Could you check a few things on this model? Use its own coordinates, in mm. Give positions to 0.01 mm unless a question says otherwise; leave off trailing zeros. Loops run counter-clockwise (first coordinate to the right, second up) from the corner with the lowest first, then second, coordinate; pieces in that order, holes last. Notation, with made-up numbers: (70, 49) - (111, 49) arc R11 ccw to (111, 59) - close; hole circle Ø8 at (-16, 79). An arc over 180 degrees is marked (long way). Write each question's results on one line, items separated by ' | '. Start each with the question number.
(1) Suppose I cut it at A-A (y = 160). Please give me the cut outline in (x, z), and give its area (3 significant figures).
(2) If we mould it in two halves opening along X, with no side actions, what happens to faces 1 (the face through (12.35, 77.07, 4.93)), 2 (the face through (99, 101, 0)), 3 (the face through (0, 99, 5)), 4 (the face through (162.86, 13.9, 4.93))? For each: released by +X, released by -X, zero draft, split by the parting line, or undercut.
(3) Suppose I cut it at C-C (y = 100). Please give me the cut outline in (x, z).
(4) Suppose I cut it at B-B (x = 13). Please give me the cut outline in (y, z), and give its area (3 significant figures).
(5) I need wall thicknesses on line 1 (Y direction, x = 160, z = 4); line 2 (Y direction, x = 13, z = 3); line 3 (Y direction, x = 186, z = 2.75). Which ranges of each line are inside material? Lowest first, please.
from build123d import *

# Parameters (mm, degrees)
SKETCH_W   = 200
SKETCH_H   = 200
SKETCH_R   = 15
SKETCH_R_2 = 3
PAD_DEPTH  = 10
FILLET_R   = 3


with BuildPart() as part:
    # Sketch → Pad (new body)
    with BuildSketch(Plane.XY):
        with Locations((100, 100)):
            Rectangle(SKETCH_W, SKETCH_H)
        with Locations((136, 100)):
            Circle(SKETCH_R, mode=Mode.SUBTRACT)
        with Locations((118.32233, 117.67767)):
            Circle(SKETCH_R_2, mode=Mode.SUBTRACT)
        with Locations((153.67767, 117.67767)):
            Circle(SKETCH_R_2, mode=Mode.SUBTRACT)
        with Locations((118.32233, 82.32233)):
            Circle(SKETCH_R_2, mode=Mode.SUBTRACT)
        with Locations((153.67767, 82.32233)):
            Circle(SKETCH_R_2, mode=Mode.SUBTRACT)
        with Locations((40, 13)):
            Circle(SKETCH_R_2, mode=Mode.SUBTRACT)
        with Locations((160, 13)):
            Circle(SKETCH_R_2, mode=Mode.SUBTRACT)
        with Locations((80, 13)):
            Circle(SKETCH_R_2, mode=Mode.SUBTRACT)
        with Locations((120, 13)):
            Circle(SKETCH_R_2, mode=Mode.SUBTRACT)
        with Locations((40, 187)):
            Circle(SKETCH_R_2, mode=Mode.SUBTRACT)
        with Locations((80, 187)):
            Circle(SKETCH_R_2, mode=Mode.SUBTRACT)
        with Locations((120, 187)):
            Circle(SKETCH_R_2, mode=Mode.SUBTRACT)
        with Locations((160, 187)):
            Circle(SKETCH_R_2, mode=Mode.SUBTRACT)
        with Locations((13, 160)):
            Circle(SKETCH_R_2, mode=Mode.SUBTRACT)
        with Locations((13, 120)):
            Circle(SKETCH_R_2, mode=Mode.SUBTRACT)
        with Locations((13, 80)):
            Circle(SKETCH_R_2, mode=Mode.SUBTRACT)
        with Locations((13, 40)):
            Circle(SKETCH_R_2, mode=Mode.SUBTRACT)
        with Locations((187, 160)):
            Circle(SKETCH_R_2, mode=Mode.SUBTRACT)
        with Locations((187, 120)):
            Circle(SKETCH_R_2, mode=Mode.SUBTRACT)
        with Locations((187, 80)):
            Circle(SKETCH_R_2, mode=Mode.SUBTRACT)
        with Locations((187, 40)):
            Circle(SKETCH_R_2, mode=Mode.SUBTRACT)
    extrude(amount=PAD_DEPTH)

    # Fillet
    fillet_edges = [part.edges().sort_by_distance(p)[0] for p in [
        (0, 0, 5),
        (200, 0, 5),
        (0, 200, 5),
        (200, 200, 5),
    ]]
    fillet(fillet_edges, radius=FILLET_R)


solid = part.part
Output values:
1) outline: (0, 0) - (10, 0) - (10, 10) - (0, 10) - close; (16, 0) - (184, 0) - (184, 10) - (16, 10) - close; (190, 0) - (200, 0) - (200, 10) - (190, 10) - close | area: 1,880 mm2
2) face 1: undercut | face 2: zero draft | face 3: released by -X | face 4: undercut
3) outline: (0, 0) - (121, 0) - (121, 10) - (0, 10) - close; (151, 0) - (200, 0) - (200, 10) - (151, 10) - close
4) outline: (0, 0) - (37, 0) - (37, 10) - (0, 10) - close; (43, 0) - (77, 0) - (77, 10) - (43, 10) - close; (83, 0) - (117, 0) - (117, 10) - (83, 10) - close; (123, 0) - (157, 0) - (157, 10) - (123, 10) - close; (163, 0) - (200, 0) - (200, 10) - (163, 10) - close | area: 1,760 mm2
5) line 1: 0 to 10, 16 to 184, 190 to 200 | line 2: 0 to 37, 43 to 77, 83 to 117, 123 to 157, 163 to 200 | line 3: 0 to 37.17, 42.83 to 77.17, 82.83 to 117.17, 122.83 to 157.17, 162.83 to 200
